The drawing under review shows one solid part. Ordinate dimensions are in mm from its lowest x, y, z. Coordinates: 2 decimals unless noted, no trailing zeros. Write each loop counter-clockwise with the first axis right and the second up, starting at its lowest first coordinate (ties: lowest second). Pieces come first, ordered by that corner, then holes.
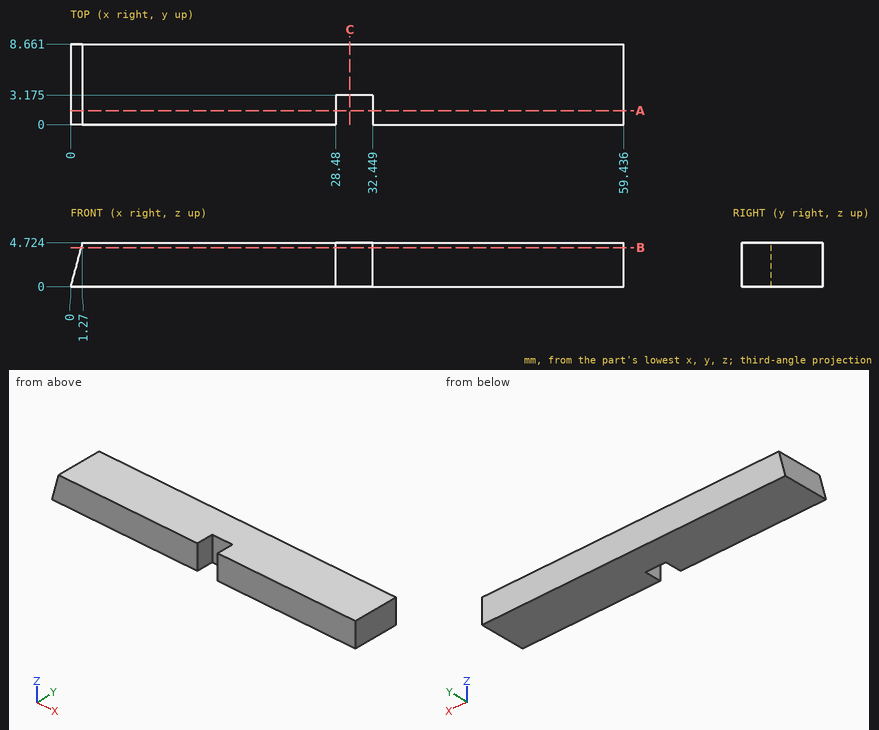
Q1. Add section B-B (z = 4.2). State the section outline as (x, y) points (1 decimal).
Ans:
outline: (1.1, 0) - (28.5, 0) - (28.5, 3.2) - (32.4, 3.2) - (32.4, 0) - (59.4, 0) - (59.4, 8.7) - (1.1, 8.7) - close
Q2. For probe 1 along X at (y, z) = (3.5, 3.35) (1 decimal); probe 2 along X at (y, z) = (6, 4.45) (1 decimal), list the stretches that pass through material, from the lowest coordinate up.
Ans:
probe 1: x = 0.9 to 59.4
probe 2: x = 1.2 to 59.4
Q3. Add section A-A (y = 1.5). State the section outline as (x, z) points (1 decimal), then the cut area to 3 significant figures.
Ans:
outline: (0, 0) - (28.5, 0) - (28.5, 4.7) - (1.3, 4.7) - close; (32.4, 0) - (59.4, 0) - (59.4, 4.7) - (32.4, 4.7) - close
area: 259 mm2
Q4. Clearance check with flat-ended pins moving along their axes: pin 1 Ø1 at (y, z) = (1, 3.5) entering from -X; pin 2 Ø1.5 at (y, z) = (5, 3.5) entering from -X. State where each tip first meets the part, or that it passes through.
Ans:
pin 1: stops at x = 0.81
pin 2: stops at x = 0.74
Q5. Add section C-C (x = 30). State the section outline as (y, z) points (1 decimal), then the cut area to 3 significant figures.
Ans:
outline: (3.2, 0) - (8.7, 0) - (8.7, 4.7) - (3.2, 4.7) - close
area: 25.9 mm2
